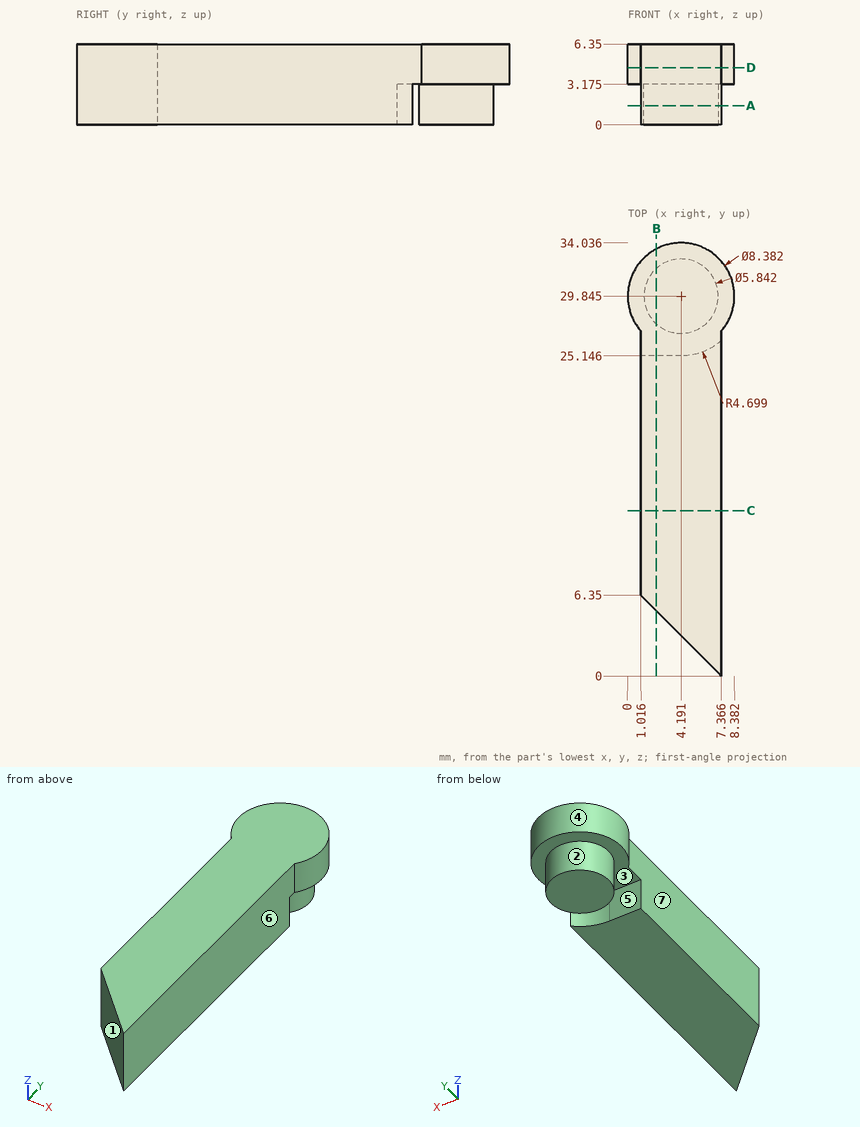
Geometry: see drawing. Coordinates: mm, zero at the bounding-box minimum. A direction names the side the tool comes from. Give positions to 0.01 mm unless a question says otherwise; leave off trailing zeros. Order: outer loops, then holes, each group sorted by start corner. A loop starts at its lowest first (then second) coordinate and runs counter-clockwise, first axis right, second up. Notation, with made-up numbers: (16.5, 57) -> (31.5, 57) arc R6 ccw to (31.5, 63) -> close; hole circle Ø3 at (41, 67). An arc over 180 degrees is marked (long way). Write each question's results on one line, items separated by ' | '. Start each with the question number.
1) Section B-B (x = 2.25). Return loops of the section in (y, z) (3 decimals), then the cut area to 3 significant figures.
2) Line query: line 1 (X direction, y = 23, z = 1.5); line 2 (Y direction, x = 2.25, z = 2); line 3 (Y direction, x = 3, z = 1.5). Output: solid intervals per line, ascending. Write a range as from..to.
3) Draft query along Y for the marked faces 1, 2, 3 and 4. Return one class per face: pulls with the +Y half, pulls with the -Y half, needs draft (parallel to the pull), parting line crosses it, or undercut.
4) Set-up query: the marked faces 5, 6 and 7. Return all of +Z, -Z, +X, -X, +Y, -Y with unobstructed straight access to the full face (end or side cutting, diameter ignored); none if empty.
5) First-contact query: pin 1 (3 mm diameter, centred on y = 14.5, z = 2.5, fed in from +X); pin 2 (2 mm diameter, centred on x = 2.5, z = 2.5, fed in from -Y); pin 3 (1 mm diameter, centred on x = 4.5, z = 1, fed in from -Y). Flat tips, straight axial feed; report the tip coordinate or a pass-through.
6) Section D-D (z = 4.5). Return loops of the section in (x, y) (3 decimals), then the cut area to 3 significant figures.
7) Section C-C (y = 13). Return loops of the section in (x, z).
8) Section A-A (z = 1.5). Return loops of the section in (x, y) (3 decimals), then the cut area to 3 significant figures.
Calculated:
1) outline: (5.116, 0) -> (25.146, 0) -> (25.146, 3.175) -> (27.662, 3.175) -> (27.662, 0) -> (32.028, 0) -> (32.028, 3.175) -> (33.559, 3.175) -> (33.559, 6.35) -> (5.116, 6.35) -> close | area: 168 mm2
2) line 1: 1.02..7.37 | line 2: 5.12..25.15, 27.66..32.03 | line 3: 4.37..25.15, 27.18..32.51
3) face 1: pulls with the -Y half | face 2: undercut | face 3: undercut | face 4: parting line crosses it
4) face 5: -Z, -X | face 6: +Z, -Z, +X, -Y | face 7: +Z, -Z, -X, -Y
5) pin 1: x = 7.37 | pin 2: y = 3.87 | pin 3: y = 2.37
6) outline: (1.016, 6.35) -> (7.366, 0) -> (7.366, 27.109) arc R4.191 ccw (long way) to (1.016, 27.109) -> close | area: 201 mm2
7) outline: (1.02, 0) -> (7.37, 0) -> (7.37, 6.35) -> (1.02, 6.35) -> close
8) outline: (1.016, 6.35) -> (7.366, 0) -> (7.366, 26.381) arc R4.699 cw to (4.191, 25.146) -> (1.016, 25.146) -> close; circle Ø5.842 at (4.191, 29.845) | area: 168 mm2
